from build123d import *

# Parameters (mm, degrees)
F0_W      = 100
F0_H      = 40
F1_DEPTH  = 2
F2_W      = 100
F2_H      = 2
F3_DEPTH  = 50
F4_W      = 100
F4_H      = 2
F5_DEPTH  = 30
F6_R      = 5
F7_DEPTH  = 100
F8_W      = 60
F8_H      = 2
F9_DEPTH  = 25
F10_W     = 60
F10_H     = 2
F11_DEPTH = 50
F12_W     = 2
F12_H     = 50
F13_DEPTH = 25


with BuildPart() as f1:
    # F0 (on Top) → F1 (new body)
    with BuildSketch(Plane.XY):
        Rectangle(F0_W, F0_H)
    extrude(amount=F1_DEPTH)

    # F2 (on face) → F3 (join)
    with BuildSketch(Plane.XY.offset(2)):
        with Locations((0, 19)):
            Rectangle(F2_W, F2_H)
    extrude(amount=F3_DEPTH)

    # F4 (on face) → F5 (join)
    with BuildSketch(Plane.XZ.offset(-18)):
        with Locations((0, 51)):
            Rectangle(F4_W, F4_H)
    extrude(amount=F5_DEPTH)

    # F6 (on face) → F7 (cut)
    with BuildSketch(Plane.XY.offset(52)):
        with Locations((30, 0)):
            Circle(F6_R)
        with Locations((-30, 0)):
            Circle(F6_R)
    extrude(amount=-F7_DEPTH, mode=Mode.SUBTRACT)

    # F8 (on face) → F9 (join)
    with BuildSketch(Plane(origin=(0, 0, 0), x_dir=(1, 0, 0), z_dir=(0, 0, -1))):
        with Locations((0, 19)):
            Rectangle(F8_W, F8_H)
    extrude(amount=F9_DEPTH)

    # F10 (on face) → F11 (join)
    with BuildSketch(Plane.XZ.offset(20)):
        with Locations((0, -24)):
            Rectangle(F10_W, F10_H)
    extrude(amount=F11_DEPTH)

    # F12 (on face) → F13 (join)
    with BuildSketch(Plane.XY.offset(-23)):
        with Locations((-29, -45)):
            Rectangle(F12_W, F12_H)
        with Locations((29, -45)):
            Rectangle(F12_W, F12_H)
    extrude(amount=F13_DEPTH)


solid = f1.part
CAD build for the part. Positions are in the model's coordinates, mm. A direction names the side the tool comes from. Round coordinates to 2 decimals unless told otherwise and drop trailing zeros. Loops run counter-clockwise (first coordinate to the right, second up) from the corner with the lowest first, then second, coordinate; pieces in that order, holes last.
(1) Cut at D-D (y = -59.5). Give the cut face in (x, z).
(2) Two-plate mould, pull along X, no slides. Class faces 1 (the flat face through (-50, 19, 24)), 2 (the flat face through (-28, -45, -11)), 3 (the flat face through (-1, 20, 26)): +X half, -X half, draft (parallel to the pull), parting line (faces both ways), or undercut.
(3) Cut at B-B (y = 12). Give the cut face in (x, z), plus the area to 3 significant figures.
(4) Cut at A-A (y = 0). Give the cut face in (x, z), plus the area to 3 significant figures.
(5) Cut at C-C (x = -42). Give the cut face in (y, z).
(6) Which spindle directions (+Z, -Z, +X, -X, +Y, -Y) get a long thin tool onto all of the face, cutting with end or side? Do faces 4 (the flat face through (-1, 18, 26)), 5 (the flat face through (0, -18, -12)), 6 (the flat face through (0, -45, -23)). Say none if no direction does.
(7) Wall check: line 1 along X through (y, z) = (-64, -4); line 2 along Y through (x, z) = (-30, 51.35); line 3 along Z through (x, y) = (1.5, -59.5). Give the ranges that are in metal, low to high.
(8) Drop flat-ended pins along their axis: pin 1 (7.5 mm diameter, centred on x = 4, z = -15, fed in from -Y); pin 2 (10 mm diameter, centred on x = -35, z = 41.5, fed in from -Y); pin 3 (1 mm diameter, centred on x = 2, z = 51, fed in from -Y); pin 4 (1 mm diameter, centred on y = 7.5, z = -1.5, fed in from -X). Give the stop position or say it passes through.
Findings below:
1. outline: (-30, -25) - (30, -25) - (30, 2) - (28, 2) - (28, -23) - (-28, -23) - (-28, 2) - (-30, 2) - close
2. face 1: -X half
2. face 2: undercut
2. face 3: draft
3. outline: (-50, 0) - (50, 0) - (50, 2) - (-50, 2) - close; (-50, 50) - (50, 50) - (50, 52) - (-50, 52) - close
3. area: 400 mm2
4. outline: (-50, 0) - (-35, 0) - (-35, 2) - (-50, 2) - close; (-50, 50) - (-35, 50) - (-35, 52) - (-50, 52) - close; (-25, 0) - (25, 0) - (25, 2) - (-25, 2) - close; (-25, 50) - (25, 50) - (25, 52) - (-25, 52) - close; (35, 0) - (50, 0) - (50, 2) - (35, 2) - close; (35, 50) - (50, 50) - (50, 52) - (35, 52) - close
4. area: 320 mm2
5. outline: (-20, 0) - (20, 0) - (20, 52) - (-12, 52) - (-12, 50) - (18, 50) - (18, 2) - (-20, 2) - close
6. face 4: +X, -X, -Y
6. face 5: -Z, +X, -X, +Y
6. face 6: +Z, -Y
7. line 1: x = -30 to -28, 28 to 30
7. line 2: y = -12 to -5, 5 to 20
7. line 3: z = -25 to -23
8. pin 1: stops at y = -20
8. pin 2: stops at y = 18
8. pin 3: stops at y = -12
8. pin 4: passes through
